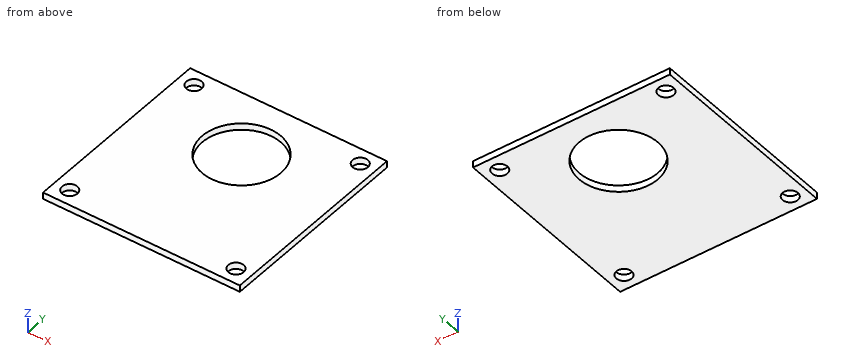
from build123d import *

# Parameters (mm, degrees)
SKETCH1_W           = 45
SKETCH1_H           = 45
BOSS_EXTRUDE1_DEPTH = 1.5
SKETCH2_R           = 1.75
SKETCH2_R_2         = 9
CUT_EXTRUDE1_DEPTH  = 32.855140872


with BuildPart() as part:
    # Sketch1 → Boss-Extrude1 (new body)
    with BuildSketch(Plane.XY):
        Rectangle(SKETCH1_W, SKETCH1_H)
    extrude(amount=BOSS_EXTRUDE1_DEPTH)

    # Sketch2 → Cut-Extrude1 (cut, through all)
    with BuildSketch(Plane.XY.offset(1.5)):
        with Locations((-19, 19)):
            Circle(SKETCH2_R)
        with Locations(Location((19, -19, 0), (0, 0, 180))):
            Circle(SKETCH2_R)
        with Locations((19, 19)):
            Circle(SKETCH2_R)
        with Locations(Location((-19, -19, 0), (0, 0, 180))):
            Circle(SKETCH2_R)
        with Locations((0, 8.1)):
            Circle(SKETCH2_R_2)
    extrude(amount=-CUT_EXTRUDE1_DEPTH, mode=Mode.SUBTRACT)


solid = part.part
Design review of the part built by this model. Coordinates are the model's own, in mm. Coordinates: 2 decimals unless noted, no trailing zeros. Order: outer loops, then holes, each group sorted by start corner. A loop starts at its lowest first (then second) coordinate and runs counter-clockwise, first axis right, second up. Notation, with made-up numbers: M 27.25,57.5 L 60.25,57.5 A36 cw 60.25,96.5 Z; hole C -29.75,80 d10. An arc over 180 degrees is marked long. Use a Markdown table: item, result.
(1) Add section C-C (z = 1.2). Give the boundary of the cut face in (x, y), then the cut area to 3 significant figures.
Worked answers:
| item | result |
|---|---|
| outline | M -22.5,-22.5 L 22.5,-22.5 L 22.5,22.5 L -22.5,22.5 Z; hole C -19,-19 d3.5; hole C -19,19 d3.5; hole C 0,8.1 d18; hole C 19,-19 d3.5; hole C 19,19 d3.5 |
| area | 1,730 mm2 |
(2) Add section D-D (x = 0). Give the boundary of the cut face in (y, z), then the cut area to 3 significant figures.
Worked answers:
| item | result |
|---|---|
| outline | M -22.5,0 L -0.9,0 L -0.9,1.5 L -22.5,1.5 Z; M 17.1,0 L 22.5,0 L 22.5,1.5 L 17.1,1.5 Z |
| area | 40.5 mm2 |
(3) Wall thickness on probe 1 along Y at (x, z) = (-19, 1.2); probe 2 along Y at (x, z) = (0, 1): over which ranges is each line inside the solid? List them lowest first.
Worked answers:
| item | result |
|---|---|
| probe 1 | y = -22.5 to -20.75, -17.25 to 17.25, 20.75 to 22.5 |
| probe 2 | y = -22.5 to -0.9, 17.1 to 22.5 |
(4) Add section A-A (x = -19). Give the boundary of the cut face in (y, z), then the cut area to 3 significant figures.
Worked answers:
| item | result |
|---|---|
| outline | M -22.5,0 L -20.75,0 L -20.75,1.5 L -22.5,1.5 Z; M -17.25,0 L 17.25,0 L 17.25,1.5 L -17.25,1.5 Z; M 20.75,0 L 22.5,0 L 22.5,1.5 L 20.75,1.5 Z |
| area | 57.0 mm2 |
